Autodesk Inventor part; units mm, degrees
ref_plane "YZ Plane" through (0, 0, 0) normal (1, 0, 0) x (0, 1, 0)
ref_plane "XZ Plane" through (0, 0, 0) normal (0, 1, 0) x (-1, 0, 0)
ref_plane "XY Plane" through (0, 0, 0) normal (0, 0, 1) x (1, 0, 0)
sketch "Sketch1" plane through (0, 0, 0) normal (1, 0, 0) x (0, 1, 0)
  circle A0 centre (0, 0) radius 60
  line L0 (0, 84) -> (0, -84) construction
  line L1 (-84, 0) -> (84, 0) construction
  dimension "d0" = 120
extrude "Flange" add sketch "Sketch1" against normal blind 7
sketch "Sketch2" plane through (0, 0, 0) normal (1, 0, 0) x (0, 0, -1)
  line L0 (-84, 0) -> (84, 0) construction
  line L1 (0, -84) -> (0, 84) construction
  point P0 (0, 0)
  point P1 (-35, 35)
  point P2 (35, 35)
  point P3 (35, -35)
  point P4 (-35, -35)
  dimension "d5" = 70
  dimension "d6" = 70
hole "Bolt Holes" at (0, 35, 35) at (0, 35, -35) at (0, -35, -35) at (0, -35, 35) direction (-1, 0, 0) diameter 8 end through all
sketch "Sketch3" plane through (-7, 0, 0) normal (-1, 0, 0) x (0, 0, 1)
  circle A0 centre (0, 0) radius 10
  dimension "d14" = 20
extrude "CV Input" add sketch "Sketch3" along normal blind 30
sketch "Sketch4" plane through (0, 0, 0) normal (1, 0, 0) x (0, 0, -1)
  circle A0 centre (0, 0) radius 35
  dimension "d20" = 70
extrude "Extrusion3" cut sketch "Sketch4" against normal blind 2
properties part number "Diff_CV_Output_V1"
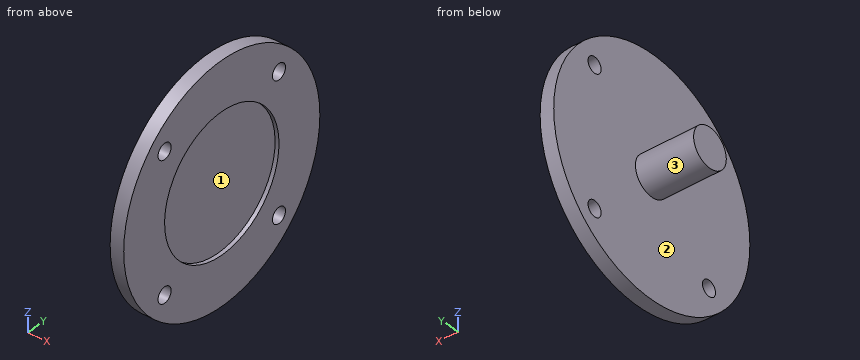
The listing builds one solid part. Answer for the finished solid, in the listing's coordinates (mm). Face numbers are marked on the shaded views. Give positions to 0.01 mm unless a question says otherwise; leave off trailing zeros. Order: outer loops, then holes, each group sorted by start corner. A loop starts at its lowest first (then second) coordinate and runs counter-clockwise, first axis right, second up. Notation, with made-up numbers: (89, 32) - (130, 32) arc R25 ccw to (130, 71) - close; hole circle Ø5 at (-28, 40). An arc over 180 degrees is marked (long way). One line per item, written item: value. Start each with the question number.
1) A cutting plane is placed at C-C on x = -31. Give the vertices of the cut face in (y, z), then the cut area to 3 significant figures.
2) A cutting plane is placed at A-A on z = 0. Give the vertices of the cut face in (x, y), then the cut area to 3 significant figures.
3) A cutting plane is placed at B-B on z = 37.5. Give the vertices of the cut face in (x, y), then the cut area to 3 significant figures.
4) The mould has two halves that part along Y. Classify the marked faces 1, 2 and 3: released by +Y, released by -Y, zero draft, split by the parting line, or undercut.
5) Find the intervals of material crossed by L1, parallel to Z at x = -3.5, y = 35; L2, parallel to X at y = -19.5, z = -26.5, in increasing order.
6) Given pin 1 Ø10.5 at (y, z) = (-35, -35) entering from -X; pin 2 Ø12 at (x, y) = (-10, 20) entering from +Z; pin 3 Ø6.5 at (y, z) = (35, -35) entering from +X; pin 4 Ø4 at (y, z) = (42.5, -7) entering from +X, each flat-ended and moving along its own axis, determine where each tip first touches the part or whether it passes through.
7) A cutting plane is placed at D-D on y = 28. Give the vertices of the cut face in (x, z), then the cut area to 3 significant figures.
Answer sheet:
1. outline: circle Ø20 at (0, 0)
1. area: 314 mm2
2. outline: (-37, -10) - (-7, -10) - (-7, -60) - (0, -60) - (0, -35) - (-2, -35) - (-2, 35) - (0, 35) - (0, 60) - (-7, 60) - (-7, 10) - (-37, 10) - close
2. area: 1,300 mm2
3. outline: (-7, -46.84) - (0, -46.84) - (0, -38.12) - (-7, -38.12) - close; (-7, -31.88) - (0, -31.88) - (0, 31.88) - (-7, 31.88) - close; (-7, 38.12) - (0, 38.12) - (0, 46.84) - (-7, 46.84) - close
3. area: 568 mm2
4. face 1: undercut
4. face 2: zero draft
4. face 3: split by the parting line
5. L1: z = -48.73 to -39, -31 to 31, 39 to 48.73
5. L2: x = -7 to -2
6. pin 1: stops at x = -7
6. pin 2: stops at z = 58.15
6. pin 3: passes through
6. pin 4: stops at x = 0
7. outline: (-7, -53.07) - (0, -53.07) - (0, -21) - (-2, -21) - (-2, 21) - (0, 21) - (0, 53.07) - (-7, 53.07) - close
7. area: 659 mm2
